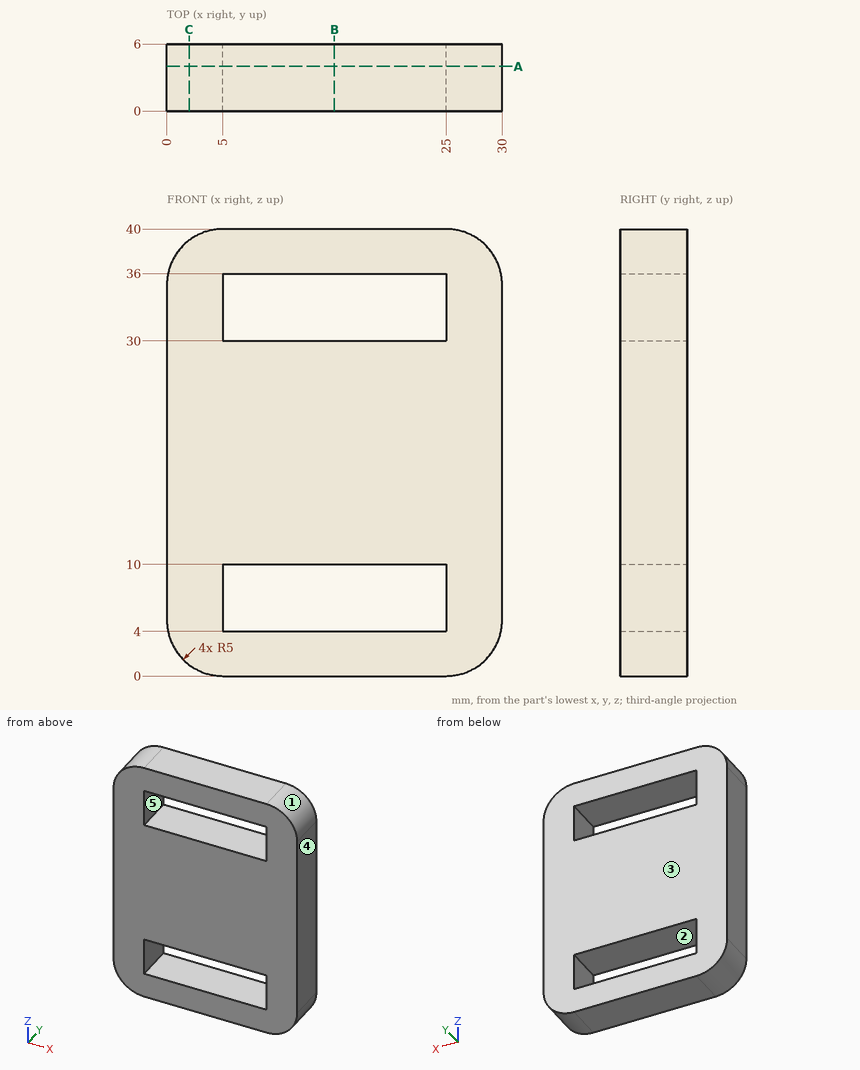
Job drawing, mm, ordinate dimensions from the low corner. One solid piece. A direction names the side the tool comes from. Round coordinates to 2 decimals unless told otherwise and drop trailing zeros. Order: outer loops, then holes, each group sorted by start corner. A loop starts at its lowest first (then second) coordinate and runs counter-clockwise, first axis right, second up. Notation, with made-up numbers: (17, 47) - (56, 47) arc R28 cw to (56, 66) - close; hole circle Ø6 at (-22, 63). An arc over 180 degrees is marked (long way). Use CSV: the item, a comma, the result in double quotes. Start each with the question number.
1) Two-plate mould, pull along Z, no slides. Class the marked faces 1, 2 and 3: pulls with the +Z half, pulls with the -Z half, needs draft (parallel to the pull), parting line crosses it, or undercut.
2) Tool access for the marked faces 4 and 5: list every direction of +Z, -Z, +X, -X, +Y, -Y with a clear straight run to the whole face (end or side of a thin tool).
3) Pin check, flat tip, straight feed: pin 1 Ø1.8 at (y, z) = (2.5, 33.5) entering from -X. Stop position of the tip, or through.
4) Saw through at C-C (x = 2). List the corners of the cut face in (y, z).
5) Wall check: L1, parallel to Z at x = 17.25, y = 0.9; L2, parallel to X at y = 2.3, z = 8; L3, parallel to X at y = 0.85, z = 36.5. Give the ranges that are in metal, low to high. Write a range as [from, to].
6) Saw through at A-A (y = 4). List the corners of the cut face in (x, z).
7) Saw through at B-B (x = 15). List the corners of the cut face in (y, z), and give its area (3 significant figures).
Values follow:
1,face 1,"pulls with the +Z half"
1,face 2,"undercut"
1,face 3,"needs draft"
2,face 4,"+Z, -Z, +X, +Y, -Y"
2,face 5,"+Y, -Y"
3,pin 1,"stops at x = 0"
4,outline,"(0, 1) - (6, 1) - (6, 39) - (0, 39) - close"
5,L1,"z = [0, 4], [10, 30], [36, 40]"
5,L2,"x = [0, 5], [25, 30]"
5,L3,"x = [0.23, 29.77]"
6,outline,"(0, 5) arc R5 ccw to (5, 0) - (25, 0) arc R5 ccw to (30, 5) - (30, 35) arc R5 ccw to (25, 40) - (5, 40) arc R5 ccw to (0, 35) - close; hole (5, 4) - (25, 4) - (25, 10) - (5, 10) - close; hole (5, 30) - (25, 30) - (25, 36) - (5, 36) - close"
7,outline,"(0, 0) - (6, 0) - (6, 4) - (0, 4) - close; (0, 10) - (6, 10) - (6, 30) - (0, 30) - close; (0, 36) - (6, 36) - (6, 40) - (0, 40) - close"
7,area,"168 mm2"
